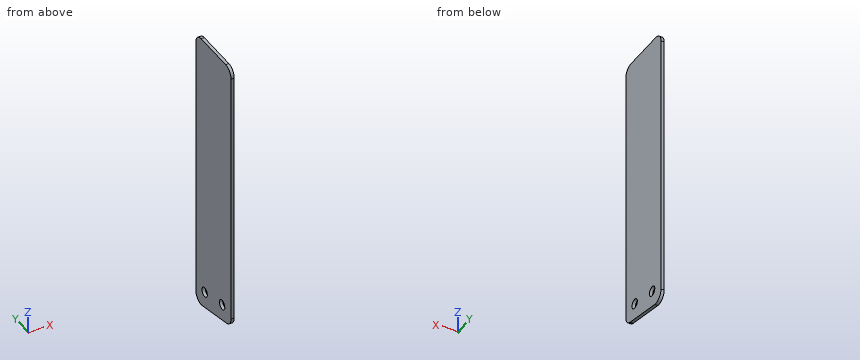
from build123d import *

# Parameters (mm, degrees)
SKETCH_1_R      = 1.5
EXTRUDE_1_DEPTH = 1
FILLET_1_R      = 3


with BuildPart() as part:
    # ｽｹｯﾁ1 → ﾎﾞｽ - 押し出し1 (new body)
    with BuildSketch(Plane(origin=(0, 0, 0), x_dir=(0, 0, -1), z_dir=(1, 0, 0))):
        Polygon((-45, 9.902902223), (-45, -9.902902223), (41.038814835, -9.902902223), (45, 9.902902223), align=None)
        with Locations((36.939800248, -4.902902223)):
            Circle(SKETCH_1_R, mode=Mode.SUBTRACT)
        with Locations((38.900973156, 4.902902223)):
            Circle(SKETCH_1_R, mode=Mode.SUBTRACT)
    extrude(amount=EXTRUDE_1_DEPTH)

    # ﾌｨﾚｯﾄ1
    fillet_1_edges = [part.edges().sort_by_distance(p)[0] for p in [
        (0.5, -9.902902223, -41.038814835),
        (0.5, -9.902902223, 45),
        (0.5, 9.902902223, 45),
        (0.5, 9.902902223, -45),
    ]]
    fillet(fillet_1_edges, radius=FILLET_1_R)


solid = part.part
Input: part model. Units: mm. Frame: model coordinates. Coordinates: 2 decimals unless noted, no trailing zeros. Loops run counter-clockwise (first coordinate to the right, second up) from the corner with the lowest first, then second, coordinate; pieces in that order, holes last. Notation, with made-up numbers: (-4.5, 86.25) -> (24.5, 86.25) arc R17 ccw to (24.5, 116.25) -> close; hole circle Ø10 at (87.5, -6). An arc over 180 degrees is marked (long way). Write item = value, one per line. Start each with the question number.
Item 1: Cut plane A-A, the plane x = 0.7. Return loops of the section in (y, z), plus the area to 3 significant figures.
Item 2: Material intervals for line 1 (Z direction, x = 0.5, y = 5); line 2 (Z direction, x = 0.6, y = -6); line 3 (Z direction, x = 0.95, y = -1), sorted ascending.
Item 3: Cut plane B-B, the plane y = -2.25. Return loops of the section in (x, z).
Item 4: First-contact query: P1, Ø1, axis at y = -6, z = 26.5, coming from the -X side. Flat tip, straight axial feed; report the tip coordinate or a pass-through.
Ans:
q1.outline = (-9.9, -38.58) arc R3 ccw to (-7.49, -41.52) -> (6.31, -44.28) arc R3 ccw to (9.9, -41.34) -> (9.9, 42) arc R3 ccw to (6.9, 45) -> (-6.9, 45) arc R3 ccw to (-9.9, 42) -> close; hole circle Ø3 at (-4.9, -36.94); hole circle Ø3 at (4.9, -38.9)
q1.area = 1,720 mm²
q2.line_1 = -44.02 to -40.4, -37.4 to 45
q2.line_2 = -41.82 to -37.96, -35.92 to 45
q2.line_3 = -42.82 to 45
q3.outline = (0, -42.57) -> (1, -42.57) -> (1, 45) -> (0, 45) -> close
q4.P1 = 0
